Source: CAD feature listing. Evaluate the final solid. Frame: model axes, mm. Face numbers are marked on the shaded views. A direction names the side the tool comes from. Coordinates: 2 decimals unless noted, no trailing zeros. Order: outer loops, then holes, each group sorted by start corner. A loop starts at its lowest first (then second) coordinate and runs counter-clockwise, first axis right, second up.
```python
from build123d import *

# Parameters (mm, degrees)
BASPROSKE_W          = 6
BASPROSKE_H          = 15
TOOTHCUT_DEPTH       = 23.045407685
TEETHCUTS_COUNT      = 28
TEETHCUTS_ANGLE      = 347.142857143
BORSKE_R             = 3
BORE_DEPTH           = 50.0000508
M4_CLEARANCE_HOLE1_D = 4.5
CIRPATTERN1_COUNT    = 4


with BuildPart() as part:
    # BasProSke → Base-Revolve (revolve)
    with BuildSketch(Plane(origin=(0, 0, 0), x_dir=(1, 0, 0), z_dir=(0, 1, 0)), mode=Mode.PRIVATE) as base_revolve_sk:
        with Locations((3, 7.5)):
            Rectangle(BASPROSKE_W, BASPROSKE_H)
    revolve(base_revolve_sk.sketch.rotate(Axis((-10, 0, 0), (1, 0, 0)), 180), axis=Axis((-10, 0, 0), (1, 0, 0)))

    # TooCutSke → ToothCut (cut, through all)
    with BuildSketch(Plane(origin=(0, 0, 0), x_dir=(0, 0, -1), z_dir=(1, 0, 0))):
        with BuildLine():
            ThreePointArc((0.471336039, 12.740284272), (0, 12.749), (-0.471336039, 12.740284272))
            ThreePointArc((-0.471336039, 12.740284272), (-0.81983923, 13.900763331), (-1.409805137, 14.959114099))
            ThreePointArc((-1.409805137, 14.959114099), (0, 15.0254), (1.409805137, 14.959114099))
            ThreePointArc((1.409805137, 14.959114099), (0.81983923, 13.900763331), (0.471336039, 12.740284272))
        make_face()
    toothcut = extrude(amount=TOOTHCUT_DEPTH, mode=Mode.SUBTRACT)

    # TeethCuts: ToothCut ×28 about axis
    teethcuts_axis = Axis((-10, 0, 0), (1, 0, 0))
    for i in range(1, TEETHCUTS_COUNT):
        add(toothcut.rotate(teethcuts_axis, i * TEETHCUTS_ANGLE / (TEETHCUTS_COUNT - 1)), mode=Mode.SUBTRACT)

    # BorSke → Bore (cut, symmetric)
    with BuildSketch(Plane(origin=(0, 0, 0), x_dir=(0, 0, -1), z_dir=(1, 0, 0))):
        with Locations(Location((0, 0, 0), (0, 0, 180))):
            Circle(BORSKE_R)
    extrude(amount=BORE_DEPTH, both=True, mode=Mode.SUBTRACT)

    # M4 Clearance Hole1 (through all)
    with Locations(Plane(origin=(6, 0, 0), x_dir=(0, 0, -1), z_dir=(1, 0, 0))):
        with Locations((0, 8)):
            m4_clearance_hole1 = Hole(M4_CLEARANCE_HOLE1_D / 2)

    # CirPattern1: M4 Clearance Hole1 ×4 about axis
    cirpattern1_axis = Axis((0, 0, 0), (1, 0, 0))
    for i in range(1, CIRPATTERN1_COUNT):
        add(m4_clearance_hole1.rotate(cirpattern1_axis, i * 360 / CIRPATTERN1_COUNT), mode=Mode.SUBTRACT)


solid = part.part
```
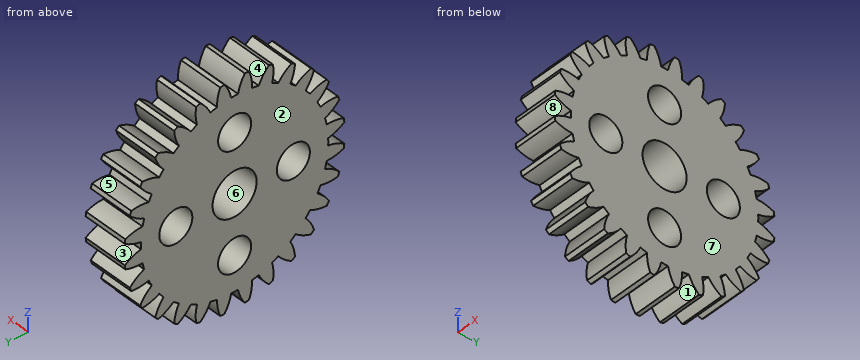
Q1. Section query D-D on z = 4.25. Output: boundary loops of the cut face in (x, y), plus the area to 3 significant figures.
Solutions:
outline: (0, -13.82) - (6, -13.82) - (6, 13.82) - (0, 13.82) - close
area: 166 mm2
Q2. Section query C-C on x = 2.2. Give the number of separate pieces and of enclosed holes in the cut face, plus the area to 3 significant figures.
Solutions:
separate pieces: 1
enclosed holes: 5
area: 509 mm2
Q3. Set-up query: the marked faces 1, 2, 3, 4 and 5. Return all of +Z, -Z, +X, -X, +Y, -Y with unobstructed straight access to the full face (end or side cutting, diameter ignored); none if empty.
Solutions:
face 1: -Z, +X, -X
face 2: +Z, -Z, -X, +Y, -Y
face 3: +X, -X, +Y
face 4: +Z, +X, -X
face 5: +X, -X
Q4. Material intervals for line 1 along Y through (x, z) = (1.3, 0); line 2 along Y through (x, z) = (1.05, 13); line 3 along Z through (x, y) = (0.9, 10.5), sorted ascending.
Solutions:
line 1: y = -12.75 to -10.25, -5.75 to -3, 3 to 5.75, 10.25 to 12.75
line 2: y = -5.3 to -3.65, -2.37 to -0.53, 0.53 to 2.37, 3.65 to 5.3
line 3: z = -10.71 to -9.59, -7.7 to 7.7, 9.59 to 10.71
Q5. Pin query (flat end, axial travel): P1, Ø1.5, axis at x = 3, z = -1.5, coming from the -Y side; P2, Ø5, axis at y = 0, z = 0, coming from the +X side. Return the tip coordinate at first contact, or that it passes through.
Solutions:
P1: stops at y = -14.94
P2: passes through
Q6. Section query A-A on z = 0. Output: boundary loops of the cut face in (x, y).
Solutions:
outline: (0, -12.75) - (6, -12.75) - (6, -10.25) - (0, -10.25) - close; (0, -5.75) - (6, -5.75) - (6, -3) - (0, -3) - close; (0, 3) - (6, 3) - (6, 5.75) - (0, 5.75) - close; (0, 10.25) - (6, 10.25) - (6, 12.75) - (0, 12.75) - close
Q7. Section query B-B on y = -7. Output: boundary loops of the cut face in (x, z), plus the area to 3 significant figures.
Solutions:
outline: (0, -12.36) - (6, -12.36) - (6, -2.02) - (0, -2.02) - close; (0, 2.02) - (6, 2.02) - (6, 12.36) - (0, 12.36) - close
area: 124 mm2
Q8. Pull-direction query (Y, two-part tool) for the marked faces 6, 7 and 8; classes: pulls with the +Y half, pulls with the -Y half, needs draft (parallel to the pull), parting line crosses it, or undercut.
Solutions:
face 6: undercut
face 7: needs draft
face 8: pulls with the -Y half
